Build history of the part. All positions in model axes, mm. A direction names the side the tool comes from. Coordinates: 2 decimals unless noted, no trailing zeros. Order: outer loops, then holes, each group sorted by start corner. A loop starts at its lowest first (then second) coordinate and runs counter-clockwise, first axis right, second up. Notation, with made-up numbers: (17, 73) - (22, 73) arc R28 ccw to (22, 95) - close; hole circle Ø6 at (54, 33.25). An arc over 180 degrees is marked (long way). One line per item, written item: value.
from build123d import *

# Parameters (mm, degrees)
F0_W      = 33.5
F0_H      = 22.5
F0_R      = 6
F1_DEPTH  = 2
F3_DEPTH  = 10
F4_W      = 6
F4_H      = 4
F5_DEPTH  = 2
F7_DEPTH  = 12
F8_W      = 6
F8_H      = 5
F9_DEPTH  = 2
F10_W     = 10
F10_H     = 2
F11_DEPTH = 5
F12_W     = 7
F12_H     = 14.5
F13_DEPTH = 2


with BuildPart() as f1:
    # F0 (on Front) → F1 (new body)
    with BuildSketch(Plane.XZ):
        with Locations((16.75, 11.25)):
            Rectangle(F0_W, F0_H)
        with Locations((16.75, 11)):
            Circle(F0_R, mode=Mode.SUBTRACT)
    extrude(amount=F1_DEPTH)

    # F2 (on face) → F3 (join)
    with BuildSketch(Plane(origin=(0, 0, 0), x_dir=(-1, 0, 0), z_dir=(0, 1, 0))):
        Polygon((-27.5, 22.5), (-33.5, 22.5), (-33.5, 0), (0, 0), (0, 22.5), (-11, 22.5), (-11, 20.5), (-2, 20.5), (-2, 2), (-31.5, 2), (-31.5, 20.5), (-27.5, 20.5), align=None)
    extrude(amount=F3_DEPTH)

    # F4 (on face) → F5 (cut, through all)
    with BuildSketch(Plane.XY.offset(22.5)):
        with Locations((8, 8)):
            Rectangle(F4_W, F4_H)
    extrude(amount=-F5_DEPTH, mode=Mode.SUBTRACT)

    # F6 (on face) → F7 (join, through all)
    with BuildSketch(Plane.XZ.offset(2)):
        with BuildLine():
            Line((33.5, 6), (33.5, 0))
            Line((33.5, 0), (35.5, 0))
            Line((35.5, 0), (35.5, 1.5))
            ThreePointArc((35.5, 1.5), (34, 3), (35.5, 4.5))
            Line((35.5, 4.5), (35.5, 6))
            Line((35.5, 6), (33.5, 6))
        make_face()
        with BuildLine():
            Line((35.5, 1.5), (35.5, 0))
            ThreePointArc((35.5, 0), (38.5, 3), (35.5, 6))
            Line((35.5, 6), (35.5, 4.5))
            ThreePointArc((35.5, 4.5), (36.56066, 4.06066), (37, 3))
            ThreePointArc((37, 3), (36.56066, 1.93934), (35.5, 1.5))
        make_face()
        with BuildLine():
            Line((0, 16.5), (0, 22.5))
            Line((0, 22.5), (-2, 22.5))
            Line((-2, 22.5), (-2, 21))
            ThreePointArc((-2, 21), (-0.93934, 20.56066), (-0.5, 19.5))
            ThreePointArc((-0.5, 19.5), (-0.93934, 18.43934), (-2, 18))
            Line((-2, 18), (-2, 16.5))
            Line((-2, 16.5), (0, 16.5))
        make_face()
        with BuildLine():
            Line((-2, 21), (-2, 22.5))
            ThreePointArc((-2, 22.5), (-5, 19.5), (-2, 16.5))
            Line((-2, 16.5), (-2, 18))
            ThreePointArc((-2, 18), (-3.5, 19.5), (-2, 21))
        make_face()
    extrude(amount=-F7_DEPTH)

    # F8 (on face) → F9 (join, through all)
    with BuildSketch(Plane.XY.offset(22.5)):
        with Locations((14, 2.5)):
            Rectangle(F8_W, F8_H)
    extrude(amount=-F9_DEPTH)

    # F10 (on face) → F11 (cut)
    with BuildSketch(Plane(origin=(0, 10, 0), x_dir=(-1, 0, 0), z_dir=(0, 1, 0))):
        with Locations((-26.5, 1)):
            Rectangle(F10_W, F10_H)
    extrude(amount=-F11_DEPTH, mode=Mode.SUBTRACT)

    # F12 (on face) → F13 (cut, through all)
    with BuildSketch(Plane(origin=(0, 0, 0), x_dir=(0, -1, 0), z_dir=(-1, 0, 0))):
        with Locations((-3.5, 9.25)):
            Rectangle(F12_W, F12_H)
    extrude(amount=-F13_DEPTH, mode=Mode.SUBTRACT)


solid = f1.part
1. Band-saw the part on C-C, the plane x = 18. Give the cut face in (y, z), and give its area (3 significant figures).
Values found:
outline: (-2, 0) - (10, 0) - (10, 2) - (0, 2) - (0, 5.13) - (-2, 5.13) - close; (-2, 16.87) - (0, 16.87) - (0, 22.5) - (-2, 22.5) - close
area: 41.5 mm2
2. Band-saw the part on D-D, the plane y = -1. Give the cut face in (x, z), and give its area (3 significant figures).
Values found:
outline: (-2, 16.5) - (0, 16.5) - (0, 0) - (35.5, 0) arc R3 ccw to (35.5, 6) - (33.5, 6) - (33.5, 22.5) - (-2, 22.5) arc R3 ccw to start; hole (-2, 18) arc R1.5 ccw to (-0.5, 19.5) arc R1.5 ccw (long way) to start; hole circle Ø12 at (16.75, 11); hole (35.5, 1.5) arc R1.5 ccw to (37, 3) arc R1.5 ccw (long way) to start
area: 679 mm2
3. Probe line 1 along Z through (x, y) = (4.5, 4); line 2 along X through (y, z) = (2, 19.75); line 3 along Z through (x, y) = (16.75, -0.9). List the from-to ranges inside material, lowest first.
Values found:
line 1: z = 0 to 2, 20.5 to 22.5
line 2: x = -4.99 to -3.48, -0.52 to 2, 31.5 to 33.5
line 3: z = 0 to 5, 17 to 22.5
4. 3-axis set-ups, long thin cutter, end or side, ignore diameter. For faces 4 (the face through (33.5, 4, 14)), 5 (the face through (8, 6, 22)), 6 (the face through (8, 4, 20.5)), 7 (the face through (27, 5, 1)): which of +Z, -Z, +X, -X, +Y, -Y reach the whole face in a straight line?
Values found:
face 4: +Z, +X, +Y, -Y
face 5: +Z, +Y
face 6: +Y
face 7: -Z, +Y
5. Two-plate mould, pull along X, no slides. Class faces 1 (the face through (19, 0, 17)), 2 (the face through (1, 10, 10)), 3 (the face through (-5, 3.9, 19.6)): pulls with the +X half, pulls with the -X half, needs draft (parallel to the pull), parting line crosses it, or undercut.
Values found:
face 1: undercut
face 2: needs draft
face 3: pulls with the -X half
6. Flat gauge pins, fed straight in: P1, Ø2, axis at x = 15, z = 21.5, coming from the +Y side; P2, Ø1.5, axis at x = 3, z = 12, coming from the +Y side; P3, Ø1.2, axis at x = 0.5, y = 5, coming from the -Z side; P4, Ø1, axis at y = 7, z = 1, coming from the +X side. Where does each tip first touch, or does it go through?
Values found:
P1: stops at y = 5
P2: stops at y = 0
P3: stops at z = 0
P4: stops at x = 38.1
7. Band-saw the part on A-A, the plane y = 8.5. Give the cut face in (x, z).
Values found:
outline: (-2, 16.5) - (0, 16.5) - (0, 0) - (21.5, 0) - (21.5, 2) - (2, 2) - (2, 20.5) - (5, 20.5) - (5, 22.5) - (-2, 22.5) arc R3 ccw to start; (27.5, 20.5) - (31.5, 20.5) - (31.5, 0) - (35.5, 0) arc R3 ccw to (35.5, 6) - (33.5, 6) - (33.5, 22.5) - (27.5, 22.5) - close; hole (-2, 18) arc R1.5 ccw to (-0.5, 19.5) arc R1.5 ccw (long way) to start; hole (35.5, 1.5) arc R1.5 ccw to (37, 3) arc R1.5 ccw (long way) to start
8. Band-saw the part on B-B, the plane z = 11. Give the cut face in (x, y).
Values found:
outline: (0, -2) - (10.75, -2) - (10.75, 0) - (0, 0) - close; (0, 7) - (2, 7) - (2, 10) - (0, 10) - close; (22.75, -2) - (33.5, -2) - (33.5, 10) - (31.5, 10) - (31.5, 0) - (22.75, 0) - close
